Build history of the part. All positions in model axes, mm. A direction names the side the tool comes from. Coordinates: 2 decimals unless noted, no trailing zeros. Order: outer loops, then holes, each group sorted by start corner. A loop starts at its lowest first (then second) coordinate and runs counter-clockwise, first axis right, second up. Notation, with made-up numbers: M 38,39 L 42,39 A10 cw 42,44 Z; hole C 48.25,-12.5 d8. An arc over 180 degrees is marked long. Write item = value, one per line. Start each with the question number.
Q1. Band-saw the part on B-B on x = 85. Write the cut outline in (y, z), plus the area to 3 significant figures.
Q2. Band-saw the part on A-A on z = -25. Write the cut outline in (x, y).
Q3. Pull direction Z, two halves, no side cores. Call faces 1 (the face through (24, 27, 0)), 2 (the face through (24, 30, -70)), 3 (the face through (76.57, 4.93, -30.38)), 4 (the face through (120, 5, -25)): released by +Z, released by -Z, zero draft, split by the parting line, or undercut.
Q4. 3-axis set-ups, long thin cutter, end or side, ignore diameter. For faces 5 (the face through (25, 40, -35)), 6 (the face through (0, 35, -35)): which of +Z, -Z, +X, -X, +Y, -Y reach the whole face in a straight line?
Q5. Drill centre lines: probe 1 along Z at (x, y) = (85, 4); probe 2 along X at (y, z) = (4, -25); probe 3 along X at (y, z) = (49.5, -41). Where is each one in solid material? Low to high.
Q6. Band-saw the part on C-C on z = -54. Write the cut outline in (x, y), plus the area to 3 significant figures.
Q7. Band-saw the part on D-D on y = 61. Write the cut outline in (x, z), plus the area to 3 significant figures.
Q8. Pin check, flat tip, straight feed: P1, Ø5, axis at y = 49.5, z = -43, coming from the +X side. Stop position of the tip, or through.
```python
from build123d import *

# Parameters (mm, degrees)
SKETCH1_W           = 120
SKETCH1_H           = 70
BOSS_EXTRUDE1_DEPTH = 10
SKETCH2_W           = 25
SKETCH2_H           = 70
BOSS_EXTRUDE2_DEPTH = 60
SKETCH3_R           = 10
CUT_EXTRUDE1_DEPTH  = 156.563491861
CHAMFER1_SIZE       = 20


with BuildPart() as part:
    # Sketch1 → Boss-Extrude1 (new body)
    with BuildSketch(Plane(origin=(0, 0, 0), x_dir=(1, 0, 0), z_dir=(0, 1, 0))):
        with Locations((60, 35)):
            Rectangle(SKETCH1_W, SKETCH1_H)
    extrude(amount=BOSS_EXTRUDE1_DEPTH)

    # Sketch2 → Boss-Extrude2 (add)
    with BuildSketch(Plane(origin=(0, 10, 0), x_dir=(1, 0, 0), z_dir=(0, 1, 0))):
        with Locations((12.5, 35)):
            Rectangle(SKETCH2_W, SKETCH2_H)
    extrude(amount=BOSS_EXTRUDE2_DEPTH)

    # Sketch3 → Cut-Extrude1 (cut, through all)
    with BuildSketch(Plane(origin=(0, 0, 0), x_dir=(1, 0, 0), z_dir=(0, 1, 0))):
        with Locations(Location((85, 25, 0), (0, 0, 90))):
            Circle(SKETCH3_R)
    extrude(amount=CUT_EXTRUDE1_DEPTH, mode=Mode.SUBTRACT)

    # Chamfer1
    chamfer1_edges = [part.edges().sort_by_distance(p)[0] for p in [
        (120, 5, -70),
    ]]
    chamfer(chamfer1_edges, length=CHAMFER1_SIZE)


solid = part.part
```
Recorded:
q1.outline = M 0,-70 L 10,-70 L 10,-35 L 0,-35 Z; M 0,-15 L 10,-15 L 10,0 L 0,0 Z
q1.area = 500 mm2
q2.outline = M 0,0 L 75,0 L 75,10 L 25,10 L 25,70 L 0,70 Z; M 95,0 L 120,0 L 120,10 L 95,10 Z
q3.face_1 = released by +Z
q3.face_2 = released by -Z
q3.face_3 = undercut
q3.face_4 = zero draft
q4.face_5 = +Z, -Z, +X, +Y
q4.face_6 = +Z, -Z, -X, +Y, -Y
q5.probe_1 = -70 to -35, -15 to 0
q5.probe_2 = 0 to 75, 95 to 120
q5.probe_3 = 0 to 25
q6.outline = M 0,0 L 116,0 L 116,10 L 25,10 L 25,70 L 0,70 Z
q6.area = 2,660 mm2
q7.outline = M 0,-70 L 25,-70 L 25,0 L 0,0 Z
q7.area = 1,750 mm2
q8.P1 = 25
